Geometry check sheet. Reference: the model listing, model coordinates, mm. Face numbers are marked on the shaded views. A direction names the side the tool comes from. Round coordinates to 2 decimals unless told otherwise and drop trailing zeros. Loops run counter-clockwise (first coordinate to the right, second up) from the corner with the lowest first, then second, coordinate; pieces in that order, holes last.
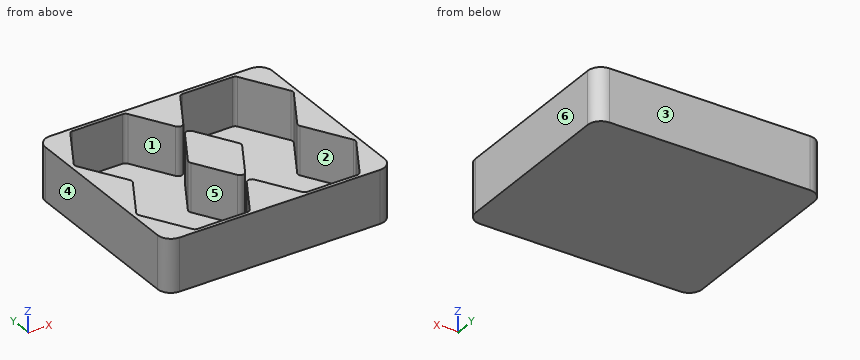
```python
from build123d import *

# Parameters (mm, degrees)
F1_DEPTH = 1
F0_W     = 51.6
F0_H     = 44.90127
F2_DEPTH = 12
F3_R     = 3
F4_R     = 1


with BuildPart() as f1:
    # F0 (on Top) → F1 (new body)
    with BuildSketch(Plane.XY):
        Polygon((18.75, 0), (25, 10.825318), (18.75, 21.650635), (6.25, 21.650635), (0, 10.825318), (-6.25, 21.650635), (-18.75, 21.650635), (-25, 10.825318), (-18.75, 0), (-25, -10.825318), (-18.75, -21.650635), (-6.25, -21.650635), (0, -10.825318), (6.25, -21.650635), (18.75, -21.650635), (25, -10.825318), align=None)
        Polygon((-6.13453, 0), (0, 10.625318), (6.13453, 0), (0, -10.625318), align=None, mode=Mode.SUBTRACT)
    extrude(amount=F1_DEPTH)

    # F0 (on Top) → F2 (join)
    with BuildSketch(Plane.XY):
        Rectangle(F0_W, F0_H)
        Polygon((18.75, 21.650635), (25, 10.825318), (18.75, 0), (25, -10.825318), (18.75, -21.650635), (6.25, -21.650635), (0, -10.825318), (-6.25, -21.650635), (-18.75, -21.650635), (-25, -10.825318), (-18.75, 0), (-25, 10.825318), (-18.75, 21.650635), (-6.25, 21.650635), (0, 10.825318), (6.25, 21.650635), align=None, mode=Mode.SUBTRACT)
        Polygon((6.13453, 0), (0, 10.625318), (-6.13453, 0), (0, -10.625318), align=None)
    extrude(amount=F2_DEPTH)

    # F3
    f3_edges = [f1.edges().sort_by_distance(p)[0] for p in [
        (25.8, -22.450635, 6),
        (25.8, 22.450635, 6),
        (-25.8, -22.450635, 6),
        (-25.8, 22.450635, 6),
    ]]
    fillet(f3_edges, radius=F3_R)

    # F4
    f4_edges = [f1.edges().sort_by_distance(p)[0] for p in [
        (0, -10.825318, 6.5),
        (0, -10.625318, 6.5),
        (6.13453, 0, 6.5),
        (0, 10.825318, 6.5),
        (0, 10.625318, 6.5),
        (-25, 10.825318, 6.5),
        (-18.75, 0, 6.5),
        (-25, -10.825318, 6.5),
        (-6.13453, 0, 6.5),
        (-18.75, -21.650635, 6.5),
        (-6.25, -21.650635, 6.5),
        (-6.25, 21.650635, 6.5),
        (-18.75, 21.650635, 6.5),
        (6.25, -21.650635, 6.5),
        (18.75, -21.650635, 6.5),
        (18.75, 0, 6.5),
        (6.25, 21.650635, 6.5),
        (18.75, 21.650635, 6.5),
        (25, 10.825318, 6.5),
        (25, -10.825318, 6.5),
    ]]
    fillet(f4_edges, radius=F4_R)


solid = f1.part
```
1) Sectioned sample at D-D, the plane y = 16. Record the cut outline in (x, z), then the cut area to 3 significant figures.
Report:
outline: (-25.8, 0) - (25.8, 0) - (25.8, 12) - (22.01, 12) - (22.01, 1) - (2.99, 1) - (2.99, 12) - (-2.99, 12) - (-2.99, 1) - (-22.01, 1) - (-22.01, 12) - (-25.8, 12) - close
area: 201 mm2
2) Sectioned sample at B-B, the plane x = 7.5. Record the cut outline in (y, z), then the cut area to 3 significant figures.
Report:
outline: (-22.45, 0) - (22.45, 0) - (22.45, 12) - (21.65, 12) - (21.65, 1) - (-21.65, 1) - (-21.65, 12) - (-22.45, 12) - close
area: 62.5 mm2
3) Sectioned sample at A-A, the plane z = 4.5. State how many separate pieces and enclosed holes the cut face has, then the cut area to 3 significant figures.
Report:
separate pieces: 2
enclosed holes: 1
area: 678 mm2
4) Sectioned sample at C-C, the plane y = 7.5. Record the cut outline in (x, z), then the cut area to 3 significant figures.
Report:
outline: (-25.8, 0) - (25.8, 0) - (25.8, 12) - (23.08, 12) - (23.08, 1) - (1.8, 1) - (1.8, 12) - (-1.8, 12) - (-1.8, 1) - (-23.08, 1) - (-23.08, 12) - (-25.8, 12) - close
area: 151 mm2
5) Access from +Z, -Z, +X, -X, +Y, -Y to the whole of each face (thin tool, end or side, straight path). Record for the marked faces 5 and 6.
Report:
face 5: +Z
face 6: +Z, -Z, +X, +Y, -Y
6) Scan lines: line 1 along Y through (x, z) = (-21.5, 8.5); line 2 along X through (y, z) = (4, 1.75); line 3 along Y through (x, z) = (1, 3.25). Record each from-to range of solid material in increasing order.
Report:
line 1: y = -22.45 to -16.89, -4.76 to 4.76, 16.89 to 22.45
line 2: x = -25.8 to -21.06, -3.83 to 3.83, 21.06 to 25.8
line 3: y = -22.45 to -12.56, -8.89 to 8.89, 12.56 to 22.45
7) Mould release check, pull along Y, two halves, no side actions. Record for the marked faces 1, 2, 3 and 4: +Y half, -Y half, draft (parallel to the pull), parting line (faces both ways), or undercut.
Report:
face 1: undercut
face 2: undercut
face 3: +Y half
face 4: draft
